Input: part model. Units: mm. Frame: model coordinates. Round coordinates to 2 decimals unless told otherwise and drop trailing zeros. Loops run counter-clockwise (first coordinate to the right, second up) from the corner with the lowest first, then second, coordinate; pieces in that order, holes last. Notation, with made-up numbers: (74.5, 15) -> (114.5, 15) arc R19 cw to (114.5, 25) -> close; hole circle Ø11 at (15.25, 30.25). An arc over 180 degrees is marked (long way). Answer in a Markdown table with one row per item. Add a question column.
Q1. Ray query, L1, parallel to X at y = 0.75, z = -4.85; L2, parallel to X at y = 1.3, z = -5.35 (3 decimals); L3, parallel to Y at x = 44, z = -7.2. Return the intervals inside material, ascending. Write a range as from..to.
Q2. Section B-B, the plane y = 0.8. Output: boundary loops of the cut face in (x, z), and give its area (3 significant figures).
Q3. Section A-A, the plane z = -4.85. Give the number of separate pieces and of enclosed holes in the cut face, and give its area (3 significant figures).
Q4. Mould query, pull axis X, two halves, no side actions, for faces 1 (the face through (7, 0, -5)), 2 (the face through (44.78, 0.99, -5.11)), 3 (the face through (-29.672, 0.986, -5.244)), 4 (the face through (-31.974, 1, -5)). Classes: pulls with the +X half, pulls with the -X half, needs draft (parallel to the pull), parting line crosses it, or undercut.
```python
from build123d import *

# Parameters (mm, degrees)
SKETCH1_W           = 80
SKETCH1_H           = 5
SKETCH1_R           = 1.5
BOSS_EXTRUDE1_DEPTH = 3
CHAMFER1_SIZE       = 1


with BuildPart() as part:
    # Sketch1 → Boss-Extrude1 (new body)
    with BuildSketch(Plane(origin=(0, 0, 0), x_dir=(1, 0, 0), z_dir=(0, 1, 0))):
        with Locations((8.025662252, 4.919288079)):
            Rectangle(SKETCH1_W, SKETCH1_H)
        with Locations(Location((-28.208163206, 4.919288079, 0), (0, 0, 270))):
            Circle(SKETCH1_R, mode=Mode.SUBTRACT)
        with Locations(Location((43.291836794, 4.919288079, 0), (0, 0, 270))):
            Circle(SKETCH1_R, mode=Mode.SUBTRACT)
    extrude(amount=BOSS_EXTRUDE1_DEPTH)

    # Chamfer1
    chamfer1_edges = [part.edges().sort_by_distance(p)[0] for p in [
        (-28.208163206, 3, -6.419288079),
        (43.291836794, 3, -6.419288079),
    ]]
    chamfer(chamfer1_edges, length=CHAMFER1_SIZE - 0.0001)  # a hair under: the kernel refuses the full size


solid = part.part
```
Answer block:
| question | item | result |
|---|---|---|
| 1 | L1 | -31.97..-29.71, -26.71..41.79, 44.79..48.03 |
| 1 | L2 | -31.974..-29.645, -26.771..41.855, 44.729..48.026 |
| 1 | L3 | 0..2.89 |
| 2 | outline | (-31.97, -7.42) -> (48.03, -7.42) -> (48.03, -2.42) -> (-31.97, -2.42) -> close; hole circle Ø3 at (-28.21, -4.92); hole circle Ø3 at (43.29, -4.92) |
| 2 | area | 386 mm^2 |
| 3 | separate pieces | 3 |
| 3 | enclosed holes | 0 |
| 3 | area | 220 mm^2 |
| 4 | face 1 | needs draft |
| 4 | face 2 | undercut |
| 4 | face 3 | undercut |
| 4 | face 4 | pulls with the -X half |
